For this review, take the finished solid that the model builds, in its own axes (mm). Coordinates: 2 decimals unless noted, no trailing zeros. Order: outer loops, then holes, each group sorted by start corner. A loop starts at its lowest first (then second) coordinate and runs counter-clockwise, first axis right, second up. Notation, with made-up numbers: (61, 88) - (100, 88) arc R16 cw to (100, 101) - close; hole circle Ø4 at (77.5, 45.25). An arc over 180 degrees is marked (long way). One line per item, written item: value. Start each with the question number.
(1) Consider section C-C on y = -164. Write out the cut boundary in (x, z), then the cut area to 3 significant figures.
(2) Consider section B-B on x = 2.5. Count the separate pieces of the cut face and the enclosed holes in it, then the cut area to 3 significant figures.
(3) Consider section A-A on y = -38.1. Write out the cut boundary in (x, z).
(4) Consider section D-D on z = 45.5. Write out the cut boundary in (x, y), then the cut area to 3 significant figures.
(5) Clearance check with flat-ended pins moving along their axes: pin 1 (5 mm diameter, centred on x = 5, z = -9.5, fed in from +Y); pin 2 (1 mm diameter, centred on x = 6.5, y = -47, fed in from +Z); pin 3 (1 mm diameter, centred on x = 6, y = -72, fed in from +Z); pin 4 (10 mm diameter, centred on y = -162.61, z = -6.84, fed in from -X). State where each tip first meets the part, or that it passes through.
(6) Mouldability with a two-part tool opening along Z and no side actions: class faces 1 (the cylindrical face through (6.261, -153.695, -24.858)), 2 (the cylindrical face through (6.26, -56.91, 24.41)), 3 (the cylindrical face through (6.261, -163.814, -12.264)) as released by +Z, released by -Z, zero draft, split by the parting line, or undercut.
(7) To check wall thickness, follow line 1 along Z through (x, y) = (2.5, 22.5); line 2 along Y through (x, z) = (7, 110); line 3 along Z through (x, y) = (3.5, -9). State the ranges of each line that lie inside material, in increasing order.
```python
from build123d import *

# Parameters (mm, degrees)
F0_R     = 5.55625
F0_R_2   = 15.875
F1_DEPTH = 12.7


with BuildPart() as f1:
    # F0 (on Right) → F1 (new body)
    with BuildSketch(Plane.YZ):
        with BuildLine():
            Line((-150.8125, -25.4), (0, -25.4))
            ThreePointArc((0, -25.4), (17.427746, -18.477923), (25.35658, -1.48454))
            Line((25.35658, -1.48454), (31.736431, 107.486081))
            ThreePointArc((31.736431, 107.486081), (25.355158, 115.736149), (16.31029, 110.54244))
            ThreePointArc((16.31029, 110.54244), (-58.360854, 23.637711), (-172.287236, 11.431516))
            ThreePointArc((-172.287236, 11.431516), (-181.366639, 7.599748), (-179.718572, -2.116315))
            Line((-179.718572, -2.116315), (-156.123724, -23.361212))
            ThreePointArc((-156.123724, -23.361212), (-153.657046, -24.872795), (-150.8125, -25.4))
        make_face()
        with Locations((-150.8125, -17.4625)):
            Circle(F0_R, mode=Mode.SUBTRACT)
        with Locations((-162.609924, -6.840052)):
            Circle(F0_R, mode=Mode.SUBTRACT)
        with Locations((-174.407348, 3.782397)):
            Circle(F0_R, mode=Mode.SUBTRACT)
        with Locations((-38.1, 0)):
            Circle(F0_R, mode=Mode.SUBTRACT)
        Circle(F0_R_2, mode=Mode.SUBTRACT)
        with Locations((23.8125, 107.95)):
            Circle(F0_R, mode=Mode.SUBTRACT)
    extrude(amount=F1_DEPTH)


solid = f1.part
```
Geometry check:
1. outline: (0, -16.27) - (12.7, -16.27) - (12.7, -12.22) - (0, -12.22) - close; (0, -1.46) - (12.7, -1.46) - (12.7, 9.38) - (0, 9.38) - close
1. area: 189 mm^2
2. separate pieces: 1
2. enclosed holes: 6
2. area: 10,300 mm^2
3. outline: (0, -25.4) - (12.7, -25.4) - (12.7, -5.56) - (0, -5.56) - close; (0, 5.56) - (12.7, 5.56) - (12.7, 36.36) - (0, 36.36) - close
4. outline: (0, -26.9) - (12.7, -26.9) - (12.7, 28.11) - (0, 28.11) - close
4. area: 699 mm^2
5. pin 1: stops at y = 24.42
5. pin 2: stops at z = 30.56
5. pin 3: stops at z = 17.5
5. pin 4: passes through
6. face 1: released by -Z
6. face 2: released by +Z
6. face 3: undercut
7. line 1: z = -11.79 to 102.55, 113.35 to 115.78
7. line 2: y = 16.12 to 18.65, 28.98 to 31.48
7. line 3: z = -25.4 to -13.08, 13.08 to 64.48
